```python
from build123d import *

# Parameters (mm, degrees)
SKETCH_1_W          = 5
SKETCH_1_H          = 120
EXTRUDE_1_DEPTH     = 80
SKETCH_2_W          = 80
SKETCH_2_H          = 5
EXTRUDE_2_DEPTH     = 150
CUT_EXTRUDE_1_REACH = 7
SKETCH_4_W          = 5
SKETCH_4_H          = 115
EXTRUDE_3_DEPTH     = 150
CUT_EXTRUDE_4_DEPTH = 2.5
CUT_EXTRUDE_5_DEPTH = 6
CUT_EXTRUDE_6_DEPTH = 6


with BuildPart() as part:
    # 草图1 → 凸台-拉伸1 (new body)
    with BuildSketch(Plane.XY):
        with Locations((2.5, -60)):
            Rectangle(SKETCH_1_W, SKETCH_1_H)
    extrude(amount=EXTRUDE_1_DEPTH)

    # 草图2 → 凸台-拉伸2 (add)
    with BuildSketch(Plane(origin=(5, 0, 0), x_dir=(0, 0, -1), z_dir=(1, 0, 0))):
        with Locations((-40, -117.5)):
            Rectangle(SKETCH_2_W, SKETCH_2_H)
    extrude(amount=EXTRUDE_2_DEPTH)

    # 草图3 → 切除-拉伸1 (cut, up to next)
    with BuildSketch(Plane(origin=(5, 0, 0), x_dir=(0, 0, -1), z_dir=(1, 0, 0)), mode=Mode.PRIVATE) as cut_extrude_1_sk1:
        with BuildLine():
            Line((-53.5, -40), (-53.5, -80))
            ThreePointArc((-53.5, -80), (-55, -81.5), (-56.5, -80))
            Line((-56.5, -80), (-56.5, -40))
            ThreePointArc((-56.5, -40), (-55, -38.5), (-53.5, -40))
        make_face()
    cut_extrude_1_tool1 = extrude(cut_extrude_1_sk1.sketch, amount=-CUT_EXTRUDE_1_REACH, mode=Mode.PRIVATE) & part.part
    add(cut_extrude_1_tool1.solids().sort_by_distance((5, -60, 55))[0], mode=Mode.SUBTRACT)
    # 草图3 → 切除-拉伸1 (cut, up to next)
    with BuildSketch(Plane(origin=(5, 0, 0), x_dir=(0, 0, -1), z_dir=(1, 0, 0)), mode=Mode.PRIVATE) as cut_extrude_1_sk2:
        with BuildLine():
            Line((-26.5, -40), (-26.5, -80))
            ThreePointArc((-26.5, -80), (-25, -81.5), (-23.5, -80))
            Line((-23.5, -80), (-23.5, -40))
            ThreePointArc((-23.5, -40), (-25, -38.5), (-26.5, -40))
        make_face()
    cut_extrude_1_tool2 = extrude(cut_extrude_1_sk2.sketch, amount=-CUT_EXTRUDE_1_REACH, mode=Mode.PRIVATE) & part.part
    add(cut_extrude_1_tool2.solids().sort_by_distance((5, -60, 25))[0], mode=Mode.SUBTRACT)
    # 草图3 → 切除-拉伸1 (cut, up to next)
    with BuildSketch(Plane(origin=(5, 0, 0), x_dir=(0, 0, -1), z_dir=(1, 0, 0)), mode=Mode.PRIVATE) as cut_extrude_1_sk3:
        with BuildLine():
            Line((-62.5, -95), (-17.5, -95))
            ThreePointArc((-17.5, -95), (-12.5, -100), (-17.5, -105))
            Line((-17.5, -105), (-62.5, -105))
            ThreePointArc((-62.5, -105), (-67.5, -100), (-62.5, -95))
        make_face()
    cut_extrude_1_tool3 = extrude(cut_extrude_1_sk3.sketch, amount=-CUT_EXTRUDE_1_REACH, mode=Mode.PRIVATE) & part.part
    add(cut_extrude_1_tool3.solids().sort_by_distance((5, -100, 40))[0], mode=Mode.SUBTRACT)

    # 草图4 → 凸台-拉伸3 (add)
    with BuildSketch(Plane(origin=(5, 0, 0), x_dir=(0, 0, -1), z_dir=(1, 0, 0))):
        with Locations((-77.5, -57.5)):
            Rectangle(SKETCH_4_W, SKETCH_4_H)
    extrude(amount=EXTRUDE_3_DEPTH)

    # 草图8 → 切除-拉伸4 (cut)
    with BuildSketch(Plane.XY.offset(80)):
        with BuildLine():
            Line((48.25, -7), (108.25, -7))
            ThreePointArc((108.25, -7), (111.25, -10), (108.25, -13))
            Line((108.25, -13), (48.25, -13))
            ThreePointArc((48.25, -13), (45.25, -10), (48.25, -7))
        make_face()
        with BuildLine():
            Line((48.25, -32), (108.25, -32))
            ThreePointArc((108.25, -32), (111.25, -29), (108.25, -26))
            Line((108.25, -26), (48.25, -26))
            ThreePointArc((48.25, -26), (45.25, -29), (48.25, -32))
        make_face()
    extrude(amount=-CUT_EXTRUDE_4_DEPTH, mode=Mode.SUBTRACT)

    # 草图6 → 切除-拉伸5 (cut, through all)
    with BuildSketch(Plane(origin=(0, 0, 75), x_dir=(-1, 0, 0), z_dir=(0, 0, -1))):
        with BuildLine():
            Line((-48.25, -11.5), (-108.25, -11.5))
            ThreePointArc((-108.25, -11.5), (-109.75, -10), (-108.25, -8.5))
            Line((-108.25, -8.5), (-48.25, -8.5))
            ThreePointArc((-48.25, -8.5), (-46.75, -10), (-48.25, -11.5))
        make_face()
        with BuildLine():
            Line((-48.25, -27.5), (-108.25, -27.5))
            ThreePointArc((-108.25, -27.5), (-109.75, -29), (-108.25, -30.5))
            Line((-108.25, -30.5), (-48.25, -30.5))
            ThreePointArc((-48.25, -30.5), (-46.75, -29), (-48.25, -27.5))
        make_face()
    extrude(amount=-CUT_EXTRUDE_5_DEPTH, mode=Mode.SUBTRACT)

    # 草图9 → 切除-拉伸6 (cut, through all)
    with BuildSketch(Plane(origin=(0, -115, 0), x_dir=(1, 0, 0), z_dir=(0, 1, 0))):
        with BuildLine():
            Line((80.25, -10), (80.25, -59))
            ThreePointArc((80.25, -59), (76.25, -63), (72.25, -59))
            Line((72.25, -59), (72.25, -10))
            ThreePointArc((72.25, -10), (76.25, -6), (80.25, -10))
        make_face()
        with BuildLine():
            Line((67.75, -5), (67.75, -65))
            ThreePointArc((67.75, -65), (66.25, -66.5), (64.75, -65))
            Line((64.75, -65), (64.75, -5))
            ThreePointArc((64.75, -5), (66.25, -3.5), (67.75, -5))
        make_face()
        with BuildLine():
            Line((88.109913979, -5), (88.109913979, -65))
            ThreePointArc((88.109913979, -65), (86.25, -66.859913979), (84.390086021, -65))
            Line((84.390086021, -65), (84.390086021, -5))
            ThreePointArc((84.390086021, -5), (86.25, -3.140086021), (88.109913979, -5))
        make_face()
    extrude(amount=-CUT_EXTRUDE_6_DEPTH, mode=Mode.SUBTRACT)


solid = part.part
```
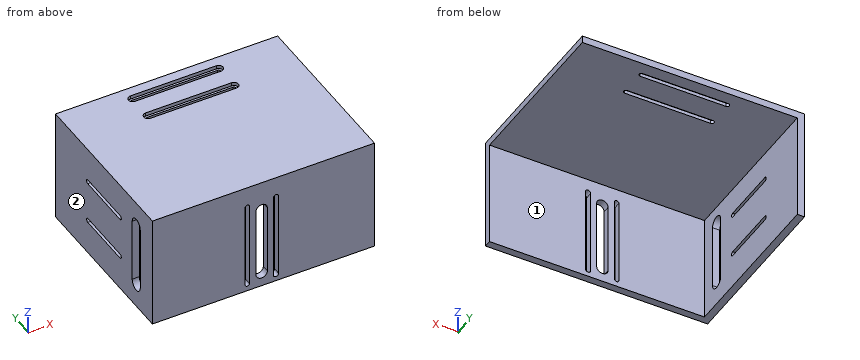
Part model, mm, in its own coordinate system. Face numbers are marked on the shaded views. A direction names the side the tool comes from. Round coordinates to 2 decimals unless told otherwise and drop trailing zeros. Write each loop counter-clockwise with the first axis right and the second up, starting at its lowest first coordinate (ties: lowest second). Pieces come first, ordered by that corner, then holes. Notation, with made-up numbers: M 26.5,64 L 39.5,64 A18 ccw 39.5,70 Z; hole C 81.5,41.5 d4. An arc over 180 degrees is marked long. One line per question, with ' | ' between items.
(1) Pin check, flat tips, straight feed: pin 1 (8 mm diameter, centred on y = -17, z = 27.5, fed in from +X); pin 2 (6 mm diameter, centred on x = 138, y = -97, fed in from -Z); pin 3 (6 mm diameter, centred on x = 100.5, z = 46, fed in from +Y). Stop position of each tip, or through.
Answer key:
pin 1: stops at x = 5 | pin 2: stops at z = 75 | pin 3: stops at y = -115
(2) 3-axis set-ups, long thin cutter, end or side, ignore diameter. For the marked faces 1 and 2: which of +Z, -Z, +X, -X, +Y, -Y reach the whole face in a straight line?
Answer key:
face 1: -Z, +X, +Y | face 2: +Z, -Z, -X, +Y, -Y
(3) Saw through at D-D on y = -20. Write the cut outline in (x, z).
Answer key:
outline: M 0,0 L 5,0 L 5,75 L 155,75 L 155,80 L 0,80 Z
(4) Saw through at C-C on z = 47.5. Write the cut outline in (x, y), then the cut area to 3 significant figures.
Answer key:
outline: M 0,-120 L 64.75,-120 L 64.75,-115 L 5,-115 L 5,-105 L 0,-105 Z; M 0,-95 L 5,-95 L 5,0 L 0,0 Z; M 67.75,-120 L 72.25,-120 L 72.25,-115 L 67.75,-115 Z; M 80.25,-120 L 84.39,-120 L 84.39,-115 L 80.25,-115 Z; M 88.11,-120 L 155,-120 L 155,-115 L 88.11,-115 Z | area: 1,230 mm^2
(5) Saw through at B-B on x = 54. Write the cut outline in (y, z).
Answer key:
outline: M -120,0 L -115,0 L -115,75 L -30.5,75 L -30.5,77.5 L -32,77.5 L -32,80 L -120,80 Z; M -27.5,75 L -11.5,75 L -11.5,77.5 L -13,77.5 L -13,80 L -26,80 L -26,77.5 L -27.5,77.5 Z; M -8.5,75 L 0,75 L 0,80 L -7,80 L -7,77.5 L -8.5,77.5 Z
(6) Saw through at A-A on x = 76.25. Write the cut outline in (y, z).
Answer key:
outline: M -120,0 L -115,0 L -115,6 L -120,6 Z; M -120,63 L -115,63 L -115,75 L -30.5,75 L -30.5,77.5 L -32,77.5 L -32,80 L -120,80 Z; M -27.5,75 L -11.5,75 L -11.5,77.5 L -13,77.5 L -13,80 L -26,80 L -26,77.5 L -27.5,77.5 Z; M -8.5,75 L 0,75 L 0,80 L -7,80 L -7,77.5 L -8.5,77.5 Z
(7) Probe line 1 along Z through (x, y) = (94, -68); line 2 along Y through (x, z) = (38, 27); line 3 along X through (y, z) = (-49.5, 73). List the from-to ranges inside material, lowest first.
Answer key:
line 1: z = 75 to 80 | line 2: y = -120 to -115 | line 3: x = 0 to 5
